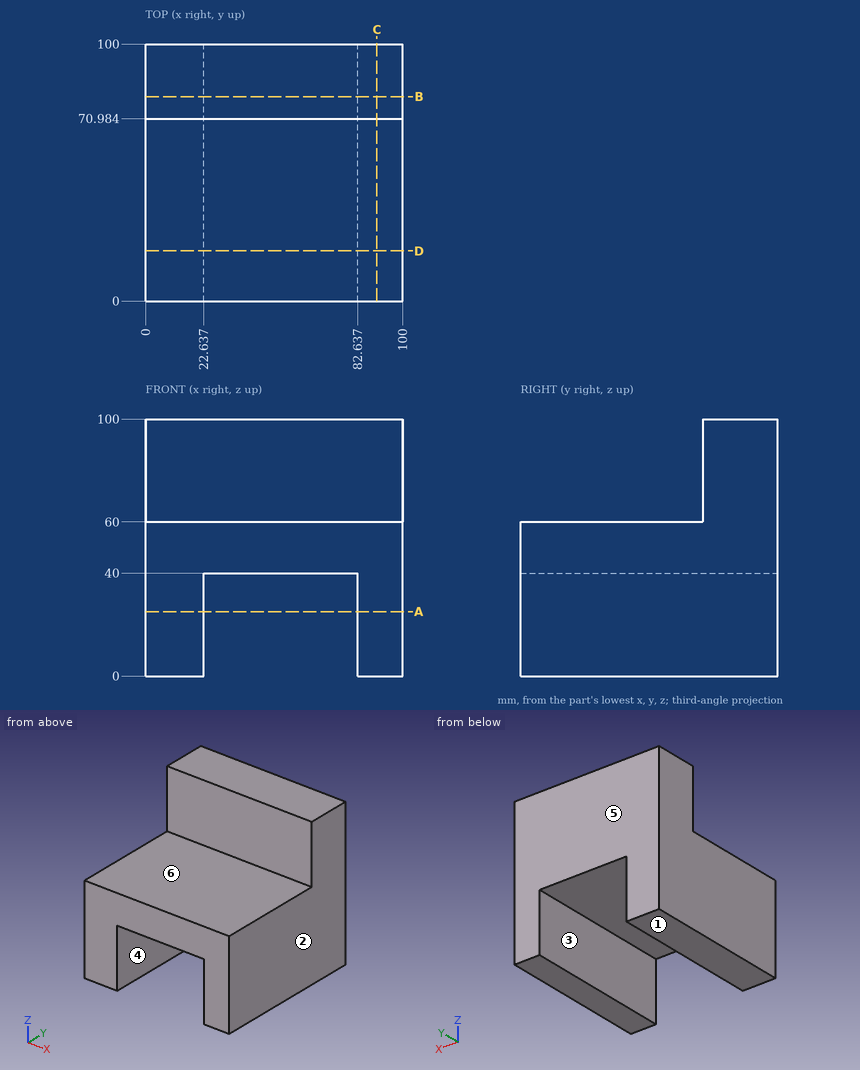
Print and shaded views of the part. All mm, measured from the part's lowest x, y and z. A direction names the side the tool comes from. Round coordinates to 2 decimals unless told otherwise and drop trailing zeros. Write each loop counter-clockwise with the first axis right and the second up, starting at its lowest first coordinate (ties: lowest second). Pieces come first, ordered by that corner, then holes. Notation, with made-up numbers: (-13, 79.25) -> (12, 79.25) arc R8 ccw to (12, 93.25) -> close; hole circle Ø6 at (73, 36.25). An arc over 180 degrees is marked (long way). Return JSON: item names as keys, results as strings. Group by question number.
Q1. Pin check, flat tips, straight feed: pin 1 (1.5 mm diameter, centred on x = 11.5, y = 27.5, fed in from +Z); pin 2 (6 mm diameter, centred on x = 33.5, y = 88, fed in from -Z); pin 3 (4 mm diameter, centred on x = 51, z = 86, fed in from -Y). Stop position of each tip, or through.
Q2. Saw through at A-A on z = 25. Write the cut outline in (x, y).
Q3. Which spindle directions (+Z, -Z, +X, -X, +Y, -Y) get a long thin tool onto all of the face, cutting with end or side? Do the marked faces 4, 5 and 6. Say none if no direction does.
Q4. Saw through at B-B on y = 79.5. Write the cut outline in (x, z).
Q5. Probe L1, parallel to X at y = 67, z = 31; L2, parallel to Z at x = 59.5, y = 42; L3, parallel to Z at x = 8, y = 37. List the from-to ranges inside material, lowest first. Write a range as [from, to].
Q6. Saw through at D-D on y = 19.5. Write the cut outline in (x, z), plus the area to 3 significant figures.
Q7. Saw through at C-C on x = 90. Write the cut outline in (y, z) (1 decimal).
Q8. Mould opens along X. For the marked faces 1, 2 and 3 say: pulls with the +X half, pulls with the -X half, needs draft (parallel to the pull), parting line crosses it, or undercut.
Answer:
{
 "1": {"pin 1": "z = 60", "pin 2": "z = 40", "pin 3": "y = 70.98"},
 "2": {"outline": "(0, 0) -> (22.64, 0) -> (22.64, 100) -> (0, 100) -> close; (82.64, 0) -> (100, 0) -> (100, 100) -> (82.64, 100) -> close"},
 "3": {"face 4": "-Z, +Y, -Y", "face 5": "+Z, -Z, +X, -X, +Y", "face 6": "+Z, +X, -X, -Y"},
 "4": {"outline": "(0, 0) -> (22.64, 0) -> (22.64, 40) -> (82.64, 40) -> (82.64, 0) -> (100, 0) -> (100, 100) -> (0, 100) -> close"},
 "5": {"L1": "[0, 22.64], [82.64, 100]", "L2": "[40, 60]", "L3": "[0, 60]"},
 "6": {"outline": "(0, 0) -> (22.64, 0) -> (22.64, 40) -> (82.64, 40) -> (82.64, 0) -> (100, 0) -> (100, 60) -> (0, 60) -> close", "area": "3,600 mm2"},
 "7": {"outline": "(0, 0) -> (100, 0) -> (100, 100) -> (71, 100) -> (71, 60) -> (0, 60) -> close"},
 "8": {"face 1": "needs draft", "face 2": "pulls with the +X half", "face 3": "undercut"}
}
